from build123d import *

# Parameters (mm, degrees)
SKETCH_1_R      = 110
SKETCH_1_R_2    = 100
SKETCH_1_R_3    = 40
SKETCH_1_R_4    = 25
SKETCH_1_R_5    = 2.1
SKETCH_1_R_6    = 10
EXTRUDE_3_DEPTH = 5
FILLET_2_R      = 5


with BuildPart() as part:
    # Эскиз1 → Бобышка-Вытянуть3 (new body)
    # profile 1 of 11: a face of its own
    with BuildSketch(Plane(origin=(0, 0, 0), x_dir=(1, 0, 0), z_dir=(0, 1, 0))):
        with Locations(Location((0, 0, 0), (0, 0, 270))):
            Circle(SKETCH_1_R)
        Circle(SKETCH_1_R_2, mode=Mode.SUBTRACT)
    # profile 2 of 11: a face of its own
    with BuildSketch(Plane(origin=(0, 0, 0), x_dir=(1, 0, 0), z_dir=(0, 1, 0))):
        with BuildLine():
            ThreePointArc((-98.875, 14.957753006), (-100, 0), (-98.875, -14.957753006))
            Line((-98.875, -14.957753006), (-39.2, -7.959899497))
            ThreePointArc((-39.2, -7.959899497), (-40, 0), (-39.2, 7.959899497))
            Line((-39.2, 7.959899497), (-98.875, 14.957753006))
        make_face()
    # profile 3 of 11: a face of its own
    with BuildSketch(Plane(origin=(0, 0, 0), x_dir=(1, 0, 0), z_dir=(0, 1, 0))):
        with BuildLine():
            ThreePointArc((-59.338454408, 80.491911572), (-70.710678119, 70.710678119), (-80.491911572, 59.338454408))
            Line((-80.491911572, 59.338454408), (-33.347084734, 22.090086911))
            ThreePointArc((-33.347084734, 22.090086911), (-28.284271247, 28.284271247), (-22.090086911, 33.347084734))
            Line((-22.090086911, 33.347084734), (-59.338454408, 80.491911572))
        make_face()
    # profile 4 of 11: a face of its own
    with BuildSketch(Plane(origin=(0, 0, 0), x_dir=(1, 0, 0), z_dir=(0, 1, 0))):
        with BuildLine():
            ThreePointArc((14.957753006, 98.875), (0, 100), (-14.957753006, 98.875))
            Line((-14.957753006, 98.875), (-7.959899497, 39.2))
            ThreePointArc((-7.959899497, 39.2), (0, 40), (7.959899497, 39.2))
            Line((7.959899497, 39.2), (14.957753006, 98.875))
        make_face()
    # profile 5 of 11: a face of its own
    with BuildSketch(Plane(origin=(0, 0, 0), x_dir=(1, 0, 0), z_dir=(0, 1, 0))):
        with BuildLine():
            Line((33.347084734, 22.090086911), (80.491911572, 59.338454408))
            ThreePointArc((80.491911572, 59.338454408), (70.710678119, 70.710678119), (59.338454408, 80.491911572))
            Line((59.338454408, 80.491911572), (22.090086911, 33.347084734))
            ThreePointArc((22.090086911, 33.347084734), (28.284271247, 28.284271247), (33.347084734, 22.090086911))
        make_face()
    # profile 6 of 11: a face of its own
    with BuildSketch(Plane(origin=(0, 0, 0), x_dir=(1, 0, 0), z_dir=(0, 1, 0))):
        with BuildLine():
            Line((39.2, -7.959899497), (98.875, -14.957753006))
            ThreePointArc((98.875, -14.957753006), (99.718353376, -7.5), (100, 0))
            ThreePointArc((100, 0), (99.718353376, 7.5), (98.875, 14.957753006))
            Line((98.875, 14.957753006), (39.2, 7.959899497))
            ThreePointArc((39.2, 7.959899497), (39.799497484, 4), (40, 0))
            ThreePointArc((40, 0), (39.799497484, -4), (39.2, -7.959899497))
        make_face()
    # profile 7 of 11: a face of its own
    with BuildSketch(Plane(origin=(0, 0, 0), x_dir=(1, 0, 0), z_dir=(0, 1, 0))):
        with BuildLine():
            Line((22.090086911, -33.347084734), (59.338454408, -80.491911572))
            ThreePointArc((59.338454408, -80.491911572), (70.710678119, -70.710678119), (80.491911572, -59.338454408))
            Line((80.491911572, -59.338454408), (33.347084734, -22.090086911))
            ThreePointArc((33.347084734, -22.090086911), (28.284271247, -28.284271247), (22.090086911, -33.347084734))
        make_face()
    # profile 8 of 11: a face of its own
    with BuildSketch(Plane(origin=(0, 0, 0), x_dir=(1, 0, 0), z_dir=(0, 1, 0))):
        with BuildLine():
            Line((-7.959899497, -39.2), (-14.957753006, -98.875))
            ThreePointArc((-14.957753006, -98.875), (0, -100), (14.957753006, -98.875))
            Line((14.957753006, -98.875), (7.959899497, -39.2))
            ThreePointArc((7.959899497, -39.2), (0, -40), (-7.959899497, -39.2))
        make_face()
    # profile 9 of 11: a face of its own
    with BuildSketch(Plane(origin=(0, 0, 0), x_dir=(1, 0, 0), z_dir=(0, 1, 0))):
        with BuildLine():
            ThreePointArc((-80.491911572, -59.338454408), (-70.710678119, -70.710678119), (-59.338454408, -80.491911572))
            Line((-59.338454408, -80.491911572), (-22.090086911, -33.347084734))
            ThreePointArc((-22.090086911, -33.347084734), (-28.284271247, -28.284271247), (-33.347084734, -22.090086911))
            Line((-33.347084734, -22.090086911), (-80.491911572, -59.338454408))
        make_face()
    # profile 10 of 11: a face of its own
    with BuildSketch(Plane(origin=(0, 0, 0), x_dir=(1, 0, 0), z_dir=(0, 1, 0))):
        Circle(SKETCH_1_R_3)
        Circle(SKETCH_1_R_4, mode=Mode.SUBTRACT)
    # profile 11 of 11: a face of its own
    with BuildSketch(Plane(origin=(0, 0, 0), x_dir=(1, 0, 0), z_dir=(0, 1, 0))):
        Circle(SKETCH_1_R_4)
        with Locations(Location((-12.727922061, 12.727922061, 0), (0, 0, 270))):
            Circle(SKETCH_1_R_5, mode=Mode.SUBTRACT)
        with Locations(Location((12.727922061, 12.727922061, 0), (0, 0, 270))):
            Circle(SKETCH_1_R_5, mode=Mode.SUBTRACT)
        with Locations(Location((18, 0, 0), (0, 0, 270))):
            Circle(SKETCH_1_R_5, mode=Mode.SUBTRACT)
        with Locations(Location((-12.727922061, -12.727922061, 0), (0, 0, 270))):
            Circle(SKETCH_1_R_5, mode=Mode.SUBTRACT)
        with Locations(Location((0, -18, 0), (0, 0, 270))):
            Circle(SKETCH_1_R_5, mode=Mode.SUBTRACT)
        with Locations(Location((-18, 0, 0), (0, 0, 270))):
            Circle(SKETCH_1_R_5, mode=Mode.SUBTRACT)
        with Locations(Location((12.727922061, -12.727922061, 0), (0, 0, 270))):
            Circle(SKETCH_1_R_5, mode=Mode.SUBTRACT)
        with Locations(Location((0, 18, 0), (0, 0, 270))):
            Circle(SKETCH_1_R_5, mode=Mode.SUBTRACT)
        with Locations(Location((0, 0, 0), (0, 0, 270))):
            Circle(SKETCH_1_R_6, mode=Mode.SUBTRACT)
    extrude(amount=EXTRUDE_3_DEPTH)

    # Скругление2
    fillet_2_edges = [part.edges().sort_by_distance(p)[0] for p in [
        (59.338454408, 2.5, 80.491911572),
        (22.090086911, 2.5, 33.347084734),
        (7.959899497, 2.5, 39.2),
        (14.957753006, 2.5, 98.875),
        (80.491911572, 2.5, 59.338454408),
        (98.875, 2.5, 14.957753006),
        (39.2, 2.5, 7.959899497),
        (33.347084734, 2.5, 22.090086911),
        (98.875, 2.5, -14.957753006),
        (80.491911572, 2.5, -59.338454408),
        (33.347084734, 2.5, -22.090086911),
        (39.2, 2.5, -7.959899497),
        (59.338454408, 2.5, -80.491911572),
        (14.957753006, 2.5, -98.875),
        (7.959899497, 2.5, -39.2),
        (22.090086911, 2.5, -33.347084734),
        (-14.957753006, 2.5, -98.875),
        (-59.338454408, 2.5, -80.491911572),
        (-22.090086911, 2.5, -33.347084734),
        (-7.959899497, 2.5, -39.2),
        (-80.491911572, 2.5, -59.338454408),
        (-98.875, 2.5, -14.957753006),
        (-39.2, 2.5, -7.959899497),
        (-33.347084734, 2.5, -22.090086911),
        (-98.875, 2.5, 14.957753006),
        (-80.491911572, 2.5, 59.338454408),
        (-33.347084734, 2.5, 22.090086911),
        (-39.2, 2.5, 7.959899497),
        (-59.338454408, 2.5, 80.491911572),
        (-14.957753006, 2.5, 98.875),
        (-7.959899497, 2.5, 39.2),
        (-22.090086911, 2.5, 33.347084734),
    ]]
    fillet(fillet_2_edges, radius=FILLET_2_R)


solid = part.part
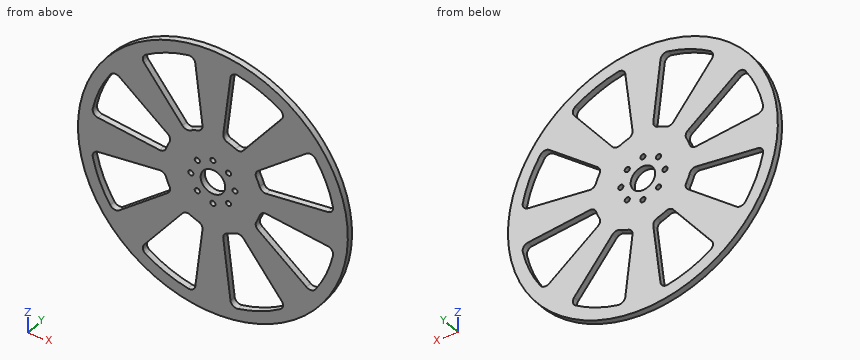
Geometry check sheet. Reference: the model listing, model coordinates, mm. Give positions to 0.01 mm unless a question says otherwise; leave off trailing zeros. Order: outer loops, then holes, each group sorted by start corner. A loop starts at its lowest first (then second) coordinate and runs counter-clockwise, first axis right, second up.
1) Cross-section at A-A (x = 50.5). Record the boundary of the cut face in (y, z) (3 decimals).
Results are:
outline: (0, -97.723) - (5, -97.723) - (5, -86.312) - (0, -86.312) - close; (0, -69.305) - (5, -69.305) - (5, -35.642) - (0, -35.642) - close; (0, -9.285) - (5, -9.285) - (5, 9.285) - (0, 9.285) - close; (0, 35.642) - (5, 35.642) - (5, 69.305) - (0, 69.305) - close; (0, 86.312) - (5, 86.312) - (5, 97.723) - (0, 97.723) - close
2) Material ranges on probe 1 along X at (y, z) = (3.3, 0); probe 2 along X at (y, z) = (4.6, -31); probe 3 along Z at (x, y) = (-78.5, 0.55), recorded low to high.
Results are:
probe 1: x = -110 to -20.1, -15.9 to -10, 10 to 15.9, 20.1 to 110
probe 2: x = -105.54 to -95.07, -44.62 to 44.62, 95.07 to 105.54
probe 3: z = -77.06 to -57.04, -12.57 to 12.57, 57.04 to 77.06
3) Gauge pin test, flat ends, axial feed: pin 1 (5.5 mm diameter, centred on x = 18, z = 0, fed in from -Y); pin 2 (2 mm diameter, centred on x = 24, y = 1.5, fed in from +Z); pin 3 (3 mm diameter, centred on y = 4, z = 58, fed in from -X); pin 4 (3 mm diameter, centred on x = -78, y = 1.5, fed in from -Z). Record the tip position at first contact, or that the pin passes through.
Results are:
pin 1: stops at y = 0
pin 2: stops at z = 107.57
pin 3: stops at x = -94.38
pin 4: stops at z = -79.04
4) Cross-section at B-B (y = 3.1). Give the number of separate pieces and of enclosed holes in the cut face, then the cut area to 3 significant figures.
Results are:
separate pieces: 1
enclosed holes: 17
area: 22,400 mm2
